Can you work these out from the model? Positions are in its coordinate system, mm. A direction names the side the tool comes from. Round coordinates to 2 decimals unless told otherwise and drop trailing zeros. Write each loop counter-clockwise with the first axis right and the second up, starting at its lowest first coordinate (ties: lowest second). Pieces come first, ordered by that corner, then holes. Notation, with made-up numbers: (2.5, 83) - (54.5, 83) arc R20 ccw to (54.5, 112) - close; hole circle Ø11 at (-16, 57.5). An arc over 180 degrees is marked (long way). One line per item, written item: value. Start each with the question number.
(1) I want a section at D-D on y = -7. List the corners of the cut face in (x, z) for me.
(2) On a 3-axis mill with a long thin cutter (end or side, diameter ignored), from which of +Z, -Z, +X, -X, +Y, -Y can I reach the whole of each face in a straight line? I mean faces 1 (the face through (5, 23, 3)), 2 (the face through (-1.003, -4.515, 1.898)), 3 (the face through (2.5, 19, 4)). Say none if no direction works.
(3) I want a section at C-C on x = -15.5. List the corners of the cut face in (y, z) for me, plus the area to 3 significant figures.
(4) Thinking about a two-plate mould opening in Y: for faces 4 (the face through (3, 31, 3)), 5 (the face through (-0.65, 24.07, 6.63)), 6 (the face through (1.88, 21.09, 3.77)), 7 (the face through (2.516, 17.786, 3.774)), which applies, +Y half, -Y half, draft (parallel to the pull), parting line (faces both ways), or undercut?
(5) If I drill on L1, parallel to X at y = 5.5, z = 4.5; L2, parallel to Y at x = 0, z = 4.75; L3, parallel to Z at x = 4, y = -12.5, over which ranges is the centre line in solid material (lowest first)? Write a range as from..to.
(6) I'm going to push flat-ended pins straight in: pin 1 Ø3 at (x, z) = (-6, 1) entering from -Y; pin 2 Ø1 at (x, z) = (-9.5, 2.5) entering from +Y; pin 3 Ø17.5 at (x, y) = (-15.5, 10) entering from +Z; pin 4 Ø5.5 at (x, y) = (0, 0) entering from +Z. Where does each tip first touch, or does it pass through?
(7) I want a section at B-B on z = 7. List the corners of the cut face in (x, y) for me.
(8) I want a section at A-A on y = 0. Give the number of separate pieces and of enclosed holes in the cut face, plus the area to 3 significant figures.
from build123d import *

# Parameters (mm, degrees)
BOSS_EXTRUDE1_DEPTH = 5.5
SKETCH2_R           = 3
BOSS_EXTRUDE2_DEPTH = 2.3
SKETCH3_R           = 3
BOSS_EXTRUDE3_DEPTH = 0.9
SKETCH4_R           = 4.625
CUT_EXTRUDE1_DEPTH  = 44.230082119
SKETCH5_R           = 1.35
CUT_EXTRUDE2_DEPTH  = 44.230082119
SKETCH7_R           = 12.35
CUT_EXTRUDE4_DEPTH  = 3.15
CUT_EXTRUDE5_DEPTH  = 3.5
SKETCH9_R           = 6.375
SKETCH9_R_2         = 4.625
BOSS_EXTRUDE4_DEPTH = 1.5
CHAMFER1_SIZE2      = 1.75
CHAMFER1_SIZE       = 1.5


with BuildPart() as part:
    # Sketch1 → Boss-Extrude1 (new body)
    with BuildSketch(Plane.XY.offset(5.5)):
        with BuildLine():
            Line((5, 18.364367672), (5, 27))
            ThreePointArc((5, 27), (2.748443387, 31.176847968), (-1.978423579, 31.591932071))
            ThreePointArc((-1.978423579, 31.591932071), (-18.536483892, 19.318360138), (-27.885598891, 0.94980064))
            ThreePointArc((-27.885598891, 0.94980064), (-27.146363183, -2.469898524), (-24, -4))
            Line((-24, -4), (-19.032866311, -4))
            ThreePointArc((-19.032866311, -4), (-15.168499178, -4.995239714), (-12.265624956, -7.733333333))
            ThreePointArc((-12.265624956, -7.733333333), (9.975316712, -10.523452689), (8.377777778, 11.834814722))
            ThreePointArc((8.377777778, 11.834814722), (5.894446616, 14.688621338), (5, 18.364367672))
        make_face()
    extrude(amount=-BOSS_EXTRUDE1_DEPTH)

    # Sketch2 → Boss-Extrude2 (add)
    with BuildSketch(Plane.XY.offset(5.5)):
        with Locations((0, 27)):
            Circle(SKETCH2_R)
    extrude(amount=BOSS_EXTRUDE2_DEPTH)

    # Sketch3 → Boss-Extrude3 (add)
    with BuildSketch(Plane.XY.offset(5.5)):
        with Locations((-24, 0)):
            Circle(SKETCH3_R)
    extrude(amount=BOSS_EXTRUDE3_DEPTH)

    # Sketch4 → Cut-Extrude1 (cut, through all)
    with BuildSketch(Plane(origin=(0, 0, 0), x_dir=(-1, 0, 0), z_dir=(0, 0, -1))):
        with Locations(Location((0, 0, 0), (0, 0, 180))):
            Circle(SKETCH4_R)
    extrude(amount=-CUT_EXTRUDE1_DEPTH, mode=Mode.SUBTRACT)

    # Sketch5 → Cut-Extrude2 (cut, through all)
    with BuildSketch(Plane.XY.offset(7.8)):
        with Locations(Location((0, 27, 0), (0, 0, 180))):
            Circle(SKETCH5_R)
        with Locations((-24, 0)):
            Circle(SKETCH5_R)
    extrude(amount=-CUT_EXTRUDE2_DEPTH, mode=Mode.SUBTRACT)

    # Sketch7 → Cut-Extrude4 (cut)
    with BuildSketch(Plane.XY.offset(5.5)):
        with Locations(Location((0, 0, 0), (0, 0, 180))):
            Circle(SKETCH7_R)
    extrude(amount=-CUT_EXTRUDE4_DEPTH, mode=Mode.SUBTRACT)

    # Sketch8 → Cut-Extrude5 (cut)
    with BuildSketch(Plane.XY.offset(5.5)):
        with BuildLine():
            Line((2.5, 18.364367672), (2.5, 19.640321115))
            ThreePointArc((2.5, 19.640321115), (1.865443882, 21.101677678), (0.364436994, 21.635721494))
            ThreePointArc((0.364436994, 21.635721494), (-2.746191158, 22.377583712), (-4.885348815, 24.754634735))
            ThreePointArc((-4.885348815, 24.754634735), (-6.159449386, 25.844240566), (-7.815189176, 25.581373906))
            ThreePointArc((-7.815189176, 25.581373906), (-16.658270057, 17.667681565), (-22.968564749, 7.617468292))
            ThreePointArc((-22.968564749, 7.617468292), (-23.002979343, 6.066010594), (-21.917514319, 4.956970002))
            ThreePointArc((-21.917514319, 4.956970002), (-21.262726036, 4.627702396), (-20.658800912, 4.212444287))
            ThreePointArc((-20.658800912, 4.212444287), (-18.994988647, 3.824188919), (-17.638370065, 4.862745371))
            ThreePointArc((-17.638370065, 4.862745371), (-10.125827676, 12.648544298), (0.431762956, 15.013758475))
            ThreePointArc((0.431762956, 15.013758475), (2.014294705, 15.621352145), (2.561932671, 17.225618165))
            ThreePointArc((2.561932671, 17.225618165), (2.5154946, 17.794151464), (2.5, 18.364367672))
        make_face()
    extrude(amount=-CUT_EXTRUDE5_DEPTH, mode=Mode.SUBTRACT)

    # Sketch9 → Boss-Extrude4 (add)
    with BuildSketch(Plane.XY.offset(2.35)):
        with Locations(Location((0, 0, 0), (0, 0, 180))):
            Circle(SKETCH9_R)
        Circle(SKETCH9_R_2, mode=Mode.SUBTRACT)
    extrude(amount=BOSS_EXTRUDE4_DEPTH)

    # Chamfer1
    chamfer1_edges = [part.edges().sort_by_distance(p)[0] for p in [
        (6.375, 0, 3.85),
    ]]
    chamfer1_side = [part.faces().sort_by_distance(p)[0] for p in [
        (6.375, 0, 3.82),
    ]]
    chamfer(chamfer1_edges, length=CHAMFER1_SIZE - 0.0001, length2=CHAMFER1_SIZE2 - 0.0001, reference=chamfer1_side[0])  # a hair under: the kernel refuses the full size


solid = part.part
Established:
1. outline: (-12.79, 0) - (12.7, 0) - (12.7, 5.5) - (10.17, 5.5) - (10.17, 2.35) - (-10.17, 2.35) - (-10.17, 5.5) - (-12.79, 5.5) - close
2. face 1: +Z, -Z, +X, +Y
2. face 2: +Z, -Z
2. face 3: +Z
3. outline: (-4.82, 0) - (22.57, 0) - (22.57, 5.5) - (18.98, 5.5) - (18.98, 2) - (8.13, 2) - (8.13, 5.5) - (-4.82, 5.5) - close
3. area: 113 mm2
4. face 4: +Y half
4. face 5: parting line
4. face 6: undercut
4. face 7: undercut
5. L1: -26.52..-22.66, -17.29..-11.06, 11.06..13.42
5. L2: -14.5..-12.35, 12.35..15.04, 21.62..25.65, 28.35..32
5. L3: 0..5.5
6. pin 1: y = -13.78
6. pin 2: y = 27.8
6. pin 3: z = 5.5
6. pin 4: through
7. outline: circle Ø6 at (0, 27); hole circle Ø2.7 at (0, 27)
8. separate pieces: 3
8. enclosed holes: 0
8. area: 125 mm2
